Check sheet for the modelled part. Datum: model origin and axes. Units: mm. Face numbers are marked on the shaded views. A direction names the side the tool comes from. Coordinates: 2 decimals unless noted, no trailing zeros. Order: outer loops, then holes, each group sorted by start corner. A loop starts at its lowest first (then second) coordinate and runs counter-clockwise, first axis right, second up.
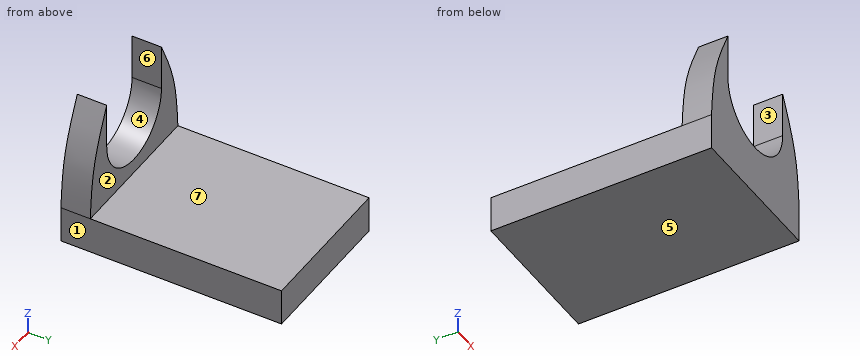
from build123d import *

# Parameters (mm, degrees)
F0_W     = 25.4
F0_H     = 38.1
F1_DEPTH = 6.35
F3_DEPTH = 5.08


with BuildPart() as f1:
    # F0 (on Top) → F1 (new body)
    with BuildSketch(Plane.XY):
        with Locations((12.7, 19.05)):
            Rectangle(F0_W, F0_H)
    extrude(amount=F1_DEPTH)

    # F2 (on face) → F3 (join)
    with BuildSketch(Plane.XZ):
        with BuildLine():
            Line((20.6375, 24.765), (20.6375, 16.8275))
            ThreePointArc((20.6375, 16.8275), (12.7, 8.89), (4.7625, 16.8275))
            Line((4.7625, 16.8275), (4.7625, 24.765))
            add(Edge.make_bspline(
                [(4.7625, 24.765), (3.3686927535, 21.8445697007), (0.6056416057, 15.9246700816), (0.1980293046, 9.5340720789), (0, 6.35)],
                knots=[0, 0, 0, 0, 0.5021426244, 1, 1, 1, 1], degree=3))
            Line((0, 6.35), (25.4, 6.35))
            add(Edge.make_bspline(
                [(20.6375, 24.765), (22.0313072465, 21.8445697007), (24.7943583943, 15.9246700816), (25.2019706954, 9.5340720789), (25.4, 6.35)],
                knots=[0, 0, 0, 0, 0.5021426244, 1, 1, 1, 1], degree=3))
        make_face()
    extrude(amount=-F3_DEPTH)


solid = f1.part
(1) Cross-section at B-B (y = 30). Enter the section's corners in (x, z).
Filled in:
outline: (0, 0) - (25.4, 0) - (25.4, 6.35) - (0, 6.35) - close
(2) Cross-section at A-A (x = 12.7). Enter the section's corners in (y, z).
Filled in:
outline: (0, 0) - (38.1, 0) - (38.1, 6.35) - (5.08, 6.35) - (5.08, 8.89) - (0, 8.89) - close
(3) Go/stop test with flat-tipped pins: P1, Ø5, axis at x = 19, z = 15.5, coming from the -Y side; P2, Ø2.5, axis at y = 2.5, z = 22.5, coming from the -X side; P3, Ø5.5, axis at y = 3, z = 21.5, coming from the +X side; P4, Ø14.5, axis at x = 16, z = 14, coming from the +Y side. Record where each tip stops, or that it passes through.
Filled in:
P1: stops at y = 0
P2: stops at x = 3.14
P3: stops at x = 23.27
P4: stops at y = 5.08
(4) Tool access check on the marked faces 5, 6 and 7. Record the directions out of +Z, -Z, +X, -X, +Y, -Y that give a thin tool (end or side, any length) a straight path to the whole face; none if there is none.
Filled in:
face 5: -Z, +X, -X, +Y, -Y
face 6: +Z, +Y, -Y
face 7: +Z, +X, -X, +Y
(5) Cross-section at C-C (x = 6). Enter the section's corners in (y, z), and give its area (3 significant figures).
Filled in:
outline: (0, 0) - (38.1, 0) - (38.1, 6.35) - (5.08, 6.35) - (5.08, 12.57) - (0, 12.57) - close
area: 274 mm2
(6) Release check for a two-part mould opening along X. For the marked faces 1, 2, 3 and 4 record: +X half, -X half, draft (parallel to the pull), parting line (faces both ways), or undercut.
Filled in:
face 1: +X half
face 2: draft
face 3: undercut
face 4: undercut
(7) Thickness scan on probe 1 along Z at (x, y) = (12.5, 32); probe 2 along Y at (x, z) = (11, 7.5); probe 3 along X at (y, z) = (5, 12.25). Record the ranges inside material, lowest first.
Filled in:
probe 1: z = 0 to 6.35
probe 2: y = 0 to 5.08
probe 3: x = 0.51 to 6.22, 19.18 to 24.89
